Geometry check sheet. Reference: drawing and pictorial views, mm from the part's lowest x, y, z. Give positions to 0.01 mm unless a question says otherwise; leave off trailing zeros. Loops run counter-clockwise (first coordinate to the right, second up) from the corner with the lowest first, then second, coordinate; pieces in that order, holes last. Notation, with made-up numbers: M 31.25,76 L 48.25,76 A33 cw 48.25,106 Z; hole C 69,73 d4. An arc over 180 degrees is marked long. One line per question, with ' | ' between items. Start each with the question number.
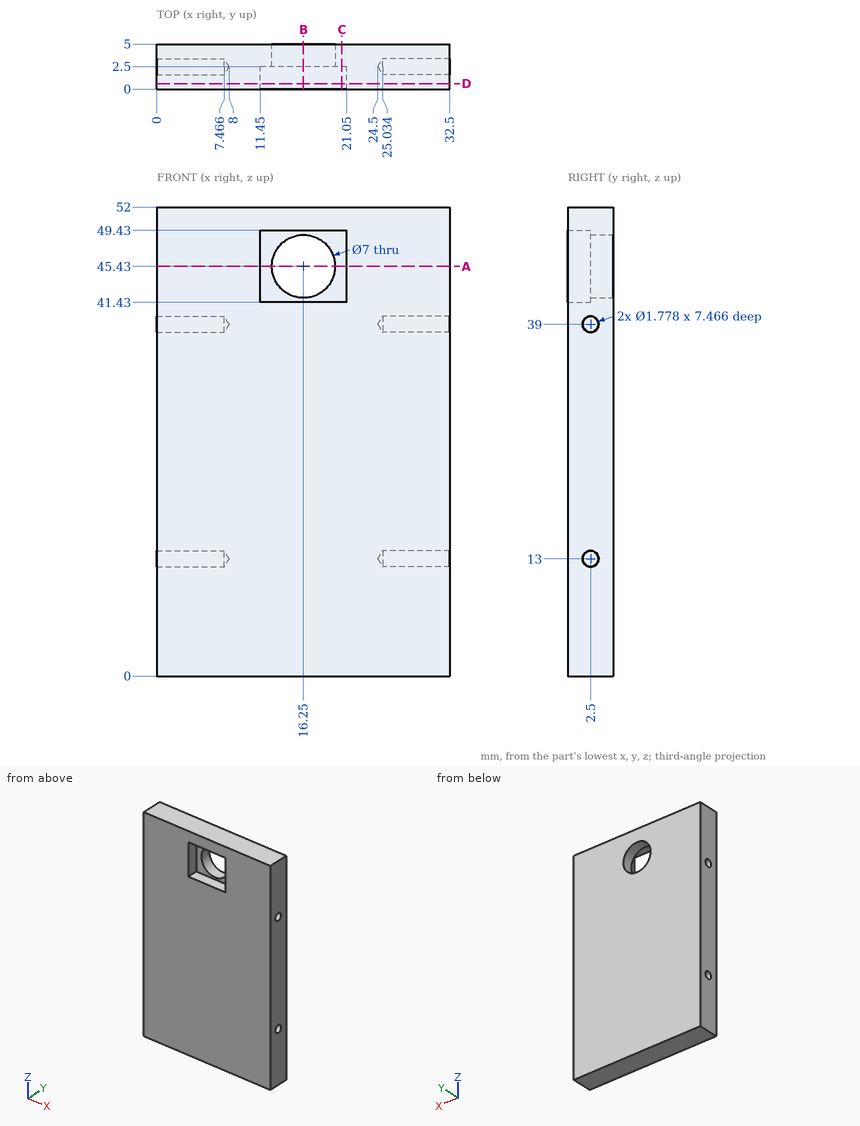
Q1. Cross-section at D-D (y = 0.6). Record the cut outline in (x, z), and give its area (3 significant figures).
Q2. Cross-section at A-A (z = 45.43). Record the cut outline in (x, y), and give its area (3 significant figures).
Q3. Cross-section at C-C (x = 20.5). Record the cut outline in (y, z), and give its area (3 significant figures).
Q4. Cross-section at B-B (x = 16.25). Record the cut outline in (y, z), and give its area (4 significant figures).
Q5. Material ranges on probe 1 along Z at (x, y) = (2.25, 2.5); probe 2 along X at (y, z) = (3.8, 45.43); probe 3 along Y at (x, z) = (4, 39), recorded low to high. Write a range as from..to.
Q6. Depth check by flat-ended pin: P1, Ø1.4, axis at y = 2.5, z = 39, coming from the +X side; P2, Ø4, axis at x = 16, z = 46.5, coming from the -Y side; P3, Ø1.4, axis at y = 2.5, z = 13, coming from the -X side. Enter the tip coordinate at first touch or a pass-through.
Solved:
1) outline: M 0,0 L 32.5,0 L 32.5,52 L 0,52 Z; hole M 11.45,41.43 L 21.05,41.43 L 21.05,49.43 L 11.45,49.43 Z | area: 1,610 mm²
2) outline: M 0,0 L 11.45,0 L 11.45,2.5 L 12.75,2.5 L 12.75,5 L 0,5 Z; M 19.75,2.5 L 21.05,2.5 L 21.05,0 L 32.5,0 L 32.5,5 L 19.75,5 Z | area: 121 mm²
3) outline: M 0,0 L 5,0 L 5,52 L 0,52 L 0,49.43 L 2.5,49.43 L 2.5,41.43 L 0,41.43 Z | area: 240 mm²
4) outline: M 0,0 L 5,0 L 5,41.93 L 2.5,41.93 L 2.5,41.43 L 0,41.43 Z; M 0,49.43 L 2.5,49.43 L 2.5,48.93 L 5,48.93 L 5,52 L 0,52 Z | area: 222.5 mm²
5) probe 1: z = 0..12.11, 13.89..38.11, 39.89..52 | probe 2: x = 0..12.75, 19.75..32.5 | probe 3: y = 0..1.61, 3.39..5
6) P1: stops at x = 24.92 | P2: passes through | P3: stops at x = 7.58
